Here's how the part is built. I have some questions about the finished solid (model axes, mm). A direction names the side the tool comes from. Coordinates: 2 decimals unless noted, no trailing zeros. Order: outer loops, then holes, each group sorted by start corner. A loop starts at its lowest first (then second) coordinate and runs counter-clockwise, first axis right, second up. Notation, with made-up numbers: (68, 87.5) -> (111, 87.5) arc R13 ccw to (111, 94.5) -> close; hole circle Ø3 at (-31, 42.25). An arc over 180 degrees is marked (long way). One line per item, written item: value. Start each with the question number.
```python
from build123d import *

# Parameters (mm, degrees)
EXTRUDE_1_DEPTH = 4.5


with BuildPart() as part:
    # 草图1 → 凸台-拉伸1 (new body)
    with BuildSketch(Plane(origin=(0, 0, 0), x_dir=(1, 0, 0), z_dir=(0, 1, 0))):
        with BuildLine():
            Line((23.680785271, 18.799740126), (23.680785271, 11.674740126))
            Line((23.680785271, 11.674740126), (19.180785271, 11.674740126))
            Line((19.180785271, 11.674740126), (19.180785271, 4.549740126))
            Line((19.180785271, 4.549740126), (23.680785271, 4.549740126))
            Line((23.680785271, 4.549740126), (23.680785271, -2.575259874))
            Line((23.680785271, -2.575259874), (19.180785271, -2.575259874))
            Line((19.180785271, -2.575259874), (19.180785271, -9.700259874))
            Line((19.180785271, -9.700259874), (23.680785271, -9.700259874))
            Line((23.680785271, -9.700259874), (23.680785271, -16.825259874))
            Line((23.680785271, -16.825259874), (19.180785271, -16.825259874))
            Line((19.180785271, -16.825259874), (19.180785271, -23.950259874))
            Line((19.180785271, -23.950259874), (23.680785271, -23.950259874))
            Line((23.680785271, -23.950259874), (23.680785271, -31.075259874))
            Line((23.680785271, -31.075259874), (19.180785271, -31.075259874))
            Line((19.180785271, -31.075259874), (19.180785271, -38.200259874))
            Line((19.180785271, -38.200259874), (8.180785271, -38.200259874))
            ThreePointArc((8.180785271, -38.200259874), (4.645251365, -36.73579378), (3.180785271, -33.200259874))
            Line((3.180785271, -33.200259874), (3.180785271, -7.200259874))
            ThreePointArc((3.180785271, -7.200259874), (0.251853083, -0.129192062), (-6.819214729, 2.799740126))
            Line((-6.819214729, 2.799740126), (-32.819214729, 2.799740126))
            ThreePointArc((-32.819214729, 2.799740126), (-36.354748635, 4.26420622), (-37.819214729, 7.799740126))
            Line((-37.819214729, 7.799740126), (-37.819214729, 18.799740126))
            Line((-37.819214729, 18.799740126), (-30.694214729, 18.799740126))
            Line((-30.694214729, 18.799740126), (-30.694214729, 23.299740126))
            Line((-30.694214729, 23.299740126), (-23.569214729, 23.299740126))
            Line((-23.569214729, 23.299740126), (-23.569214729, 18.799740126))
            Line((-23.569214729, 18.799740126), (-16.444214729, 18.799740126))
            Line((-16.444214729, 18.799740126), (-16.444214729, 23.299740126))
            Line((-16.444214729, 23.299740126), (-9.319214729, 23.299740126))
            Line((-9.319214729, 23.299740126), (-9.319214729, 18.799740126))
            Line((-9.319214729, 18.799740126), (-2.194214729, 18.799740126))
            Line((-2.194214729, 18.799740126), (-2.194214729, 23.299740126))
            Line((-2.194214729, 23.299740126), (4.930785271, 23.299740126))
            Line((4.930785271, 23.299740126), (4.930785271, 18.799740126))
            Line((4.930785271, 18.799740126), (12.055785271, 18.799740126))
            Line((12.055785271, 18.799740126), (12.055785271, 23.299740126))
            Line((12.055785271, 23.299740126), (19.180785271, 23.299740126))
            Line((19.180785271, 23.299740126), (19.180785271, 18.799740126))
            Line((19.180785271, 18.799740126), (23.680785271, 18.799740126))
        make_face()
    extrude(amount=EXTRUDE_1_DEPTH)


solid = part.part
```
Q1. I need wall thicknesses on line 1 (X direction, y = 1.4, z = -21); line 2 (Z direction, x = -31.5, y = 2); line 3 (X direction, y = 3, z = 33). Which ranges of each line are inside material? Lowest first, please.
Q2. If we mould it in two halves opening along Z, with no side actions, what happens to faces 6 (the face through (12.056, 2, -21)), 7 (the face through (19.181, 2, 6)), 8 (the face through (21, 2, -11.675)), 9 (the face through (-20, 2, -18.8))? For each: +Z half, -Z half, draft (parallel to the pull), parting line (faces both ways), or undercut.
Q3. Imagine slicing it at A-A (x = 20). Write out the boundary of the cut face in (y, z), plus the area to 3 significant figures.
Q4. Imagine slicing it at B-B (z = -10). Write out the boundary of the cut face in (x, y), plus the area to 4 significant figures.
Q5. For P1, Ø2, axis at x = 21.5, y = 2, coming from the -Z side; P2, Ø2, axis at y = 1.5, z = -20.5, coming from the +X side; P3, Ø1, axis at y = 3.5, z = 30.5, coming from the -X side, each with a flat end and sliding along its axis, tell me the tip position at first contact or that it passes through.
Q6. For faces 1 (the face through (21, 2, 9.7)), 2 (the face through (14, 2, 38.2)), 3 (the face through (-30.694, 2, -21)), 4 (the face through (-27, 2, -23.3)), 5 (the face through (-16.444, 2, -21)), which set-ups out of +Z, -Z, +X, -X, +Y, -Y let a thin tool reach every point of the face, with its end or its side?
Q7. Imagine slicing it at C-C (x = -24.5). Write out the boundary of the cut face in (y, z), plus the area to 4 significant figures.
Completed:
1. line 1: x = -30.69 to -23.57, -16.44 to -9.32, -2.19 to 4.93, 12.06 to 19.18
1. line 2: z = -18.8 to -2.8
1. line 3: x = 3.18 to 19.18
2. face 6: draft
2. face 7: undercut
2. face 8: undercut
2. face 9: -Z half
3. outline: (0, -18.8) -> (4.5, -18.8) -> (4.5, -11.67) -> (0, -11.67) -> close; (0, -4.55) -> (4.5, -4.55) -> (4.5, 2.58) -> (0, 2.58) -> close; (0, 9.7) -> (4.5, 9.7) -> (4.5, 16.83) -> (0, 16.83) -> close; (0, 23.95) -> (4.5, 23.95) -> (4.5, 31.08) -> (0, 31.08) -> close
3. area: 128 mm2
4. outline: (-37.82, 0) -> (19.18, 0) -> (19.18, 4.5) -> (-37.82, 4.5) -> close
4. area: 256.5 mm2
5. P1: stops at z = -18.8
5. P2: stops at x = 19.18
5. P3: stops at x = 3.18
6. face 1: +X, +Y, -Y
6. face 2: +Z, +X, -X, +Y, -Y
6. face 3: -Z, -X, +Y, -Y
6. face 4: -Z, +X, -X, +Y, -Y
6. face 5: -Z, +Y, -Y
7. outline: (0, -23.3) -> (4.5, -23.3) -> (4.5, -2.8) -> (0, -2.8) -> close
7. area: 92.25 mm2
